```python
from build123d import *
from build123d.topology import SkipClean

# Parameters (mm, degrees)
SKETCH2_W                           = 45
SKETCH2_H                           = 59.874368671
MAIN_EXTRUDE_DEPTH                  = 3
BOWDEN_HOLE_D                       = 4
SKETCH7_R                           = 3.5
SPACER_PILLARS_DEPTH                = 22.1
TOP_THREADS_D                       = 2.5
TOP_THREADS_DEPTH                   = 10
TOP_THREADS_TIP                     = 0.751075774
TOP_THROUGH_HOLE_D                  = 3.2
SKETCH28_R                          = 12.7
SKETCH28_R_2                        = 2
BOSS_EXTRUDE3_DEPTH                 = 2
CHUBE_MOUNTING_D                    = 3.2
CHUBE_MOUNTING_CSINK_D              = 6.72
CHUBE_MOUNTING_CSINK_ANGLE          = 90
BOSS_EXTRUDE4_DEPTH                 = 2
CARRIAGE_HOLES_D                    = 3.2
CARRIAGE_HOLES_DEPTH                = 8
CARRIAGE_HOLES_CSINK_D              = 6.72
CARRIAGE_HOLES_CSINK_ANGLE          = 90
CARRIAGE_HOLES_TIP                  = 0.96137699
BEACON_SLM_SUPPORT_HOLES_AT_2_COUNT = 2
BEACON_SLM_SUPPORT_HOLES_AT_2_PITCH = 24.748737342
BEACON_SLM_SUPPORT_HOLES_AT_3_COUNT = 2
BEACON_SLM_SUPPORT_HOLES_AT_3_PITCH = 24.748737342


with BuildPart() as part:
    # Sketch2 → Main Extrude (new body)
    with BuildSketch(Plane(origin=(0, 0, 0), x_dir=(1, 0, 0), z_dir=(0, 1, 0))):
        with Locations((-6.625631329, 14.062815665)):
            Rectangle(SKETCH2_W, SKETCH2_H)
    extrude(amount=MAIN_EXTRUDE_DEPTH)

    # Bowden Hole (through all)
    with Locations(Plane(origin=(0, 3, 0), x_dir=(1, 0, 0), z_dir=(0, 1, 0))):
        with Locations((0, 0)):
            Hole(BOWDEN_HOLE_D / 2)

    # Sketch7 → Spacer Pillars (add)
    with BuildSketch(Plane(origin=(0, 3, 0), x_dir=(1, 0, 0), z_dir=(0, 1, 0))):
        with Locations(Location((-25.625631329, 40.5, 0), (0, 0, 90))):
            Circle(SKETCH7_R)
        with Locations(Location((12.374368671, 40.5, 0), (0, 0, 90))):
            Circle(SKETCH7_R)
        with Locations(Location((-19.761284896, -2.993325275, 0), (0, 0, 90))):
            Circle(SKETCH7_R)
        with Locations(Location((12.374368671, -12.374368671, 0), (0, 0, 270))):
            Circle(SKETCH7_R)
    extrude(amount=SPACER_PILLARS_DEPTH)

    # Top Threads
    with Locations(Plane(origin=(0, 25.1, 0), x_dir=(1, 0, 0), z_dir=(0, 1, 0))):
        with Locations((12.374368671, 40.5), (-19.761284896, -2.993325275), (-25.625631329, 40.5)):
            Hole(TOP_THREADS_D / 2, depth=TOP_THREADS_DEPTH)
            with Locations((0, 0, -(TOP_THREADS_DEPTH + TOP_THREADS_TIP / 2))):  # 118° drill point
                Cone(0, TOP_THREADS_D / 2, TOP_THREADS_TIP, mode=Mode.SUBTRACT)

    # Top Through Hole (through all)
    with Locations(Plane(origin=(0, 25.1, 0), x_dir=(1, 0, 0), z_dir=(0, 1, 0))):
        with Locations((12.374368671, -12.374368671)):
            Hole(TOP_THROUGH_HOLE_D / 2)

    # Sketch28 → Boss-Extrude3 (add)
    with SkipClean():  # the faces are left unmerged after this step: merging them gives an invalid solid
        with BuildSketch(Plane(origin=(0, 3, 0), x_dir=(1, 0, 0), z_dir=(0, 1, 0))):
            with Locations(Location((0, 0, 0), (0, 0, 90))):
                Circle(SKETCH28_R)
            with Locations(Location((0, 0, 0), (0, 0, 270))):
                Circle(SKETCH28_R_2, mode=Mode.SUBTRACT)
        extrude(amount=BOSS_EXTRUDE3_DEPTH)

    # Chube Mounting (through all)
    with Locations(Plane(origin=(0, 5, 0), x_dir=(1, 0, 0), z_dir=(0, 1, 0))):
        with Locations((-4.5, 7.794228634), (4.5, 7.794228634), (9, 0), (4.5, -7.794228634), (-4.5, -7.794228634), (-9, 0)):
            CounterSinkHole(CHUBE_MOUNTING_D / 2, CHUBE_MOUNTING_CSINK_D / 2, counter_sink_angle=CHUBE_MOUNTING_CSINK_ANGLE)

    # Sketch29 → Boss-Extrude4 (add)
    with SkipClean():  # the faces are left unmerged after this step: merging them gives an invalid solid
        with BuildSketch(Plane(origin=(0, 3, 0), x_dir=(1, 0, 0), z_dir=(0, 1, 0))):
            with BuildLine():
                Line((-17.181637577, 40.5), (-17.181637577, 20.5))
                ThreePointArc((-17.181637577, 20.5), (-16.156511311, 18.025126266), (-13.681637577, 17))
                Line((-13.681637577, 17), (1.318362423, 17))
                ThreePointArc((1.318362423, 17), (3.793236157, 18.025126266), (4.818362423, 20.5))
                Line((4.818362423, 20.5), (4.818362423, 40.5))
                ThreePointArc((4.818362423, 40.5), (3.793236157, 42.974873734), (1.318362423, 44))
                Line((1.318362423, 44), (-13.681637577, 44))
                ThreePointArc((-13.681637577, 44), (-16.156511311, 42.974873734), (-17.181637577, 40.5))
            make_face()
        extrude(amount=BOSS_EXTRUDE4_DEPTH)

    # Carriage Holes
    with Locations(Plane(origin=(0, 5, 0), x_dir=(1, 0, 0), z_dir=(0, 1, 0))):
        with Locations((1.318362423, 40.5), (1.318362423, 20.5), (-13.681637577, 20.5), (-13.681637577, 40.5)):
            CounterSinkHole(CARRIAGE_HOLES_D / 2, CARRIAGE_HOLES_CSINK_D / 2, depth=CARRIAGE_HOLES_DEPTH, counter_sink_angle=CARRIAGE_HOLES_CSINK_ANGLE)
            with Locations((0, 0, -(CARRIAGE_HOLES_DEPTH + CARRIAGE_HOLES_TIP / 2))):  # 118° drill point
                Cone(0, CARRIAGE_HOLES_D / 2, CARRIAGE_HOLES_TIP, mode=Mode.SUBTRACT)

    # Sketch25 → Beacon SLM Support Holes (revolve, cut)
    with SkipClean():  # the faces are left unmerged after this step: merging them gives an invalid solid
        with BuildSketch(Plane(origin=(-12.374368671, 3, -12.374368671), x_dir=(0, 0, 1), z_dir=(1, 0, 0))):
            Polygon((0, 0), (0, 3), (1.6, 3), (1.6, 1.76), (3.36, 0), align=None)
        beacon_slm_support_holes = revolve(axis=Axis((-12.374368671, 9.35, -12.374368671), (0, -1, 0)), mode=Mode.SUBTRACT)

    # Beacon SLM Support Holes at 2: Beacon SLM Support Holes ×2
    with SkipClean():  # the faces are left unmerged after this step: merging them gives an invalid solid
        with Locations(*[(i * BEACON_SLM_SUPPORT_HOLES_AT_2_PITCH, 0, 0) for i in range(1, BEACON_SLM_SUPPORT_HOLES_AT_2_COUNT)]):
            add(beacon_slm_support_holes, mode=Mode.SUBTRACT)

    # Beacon SLM Support Holes at 3: Beacon SLM Support Holes ×2
    with SkipClean():  # the faces are left unmerged after this step: merging them gives an invalid solid
        with Locations(*[(0, 0, i * BEACON_SLM_SUPPORT_HOLES_AT_3_PITCH) for i in range(1, BEACON_SLM_SUPPORT_HOLES_AT_3_COUNT)]):
            add(beacon_slm_support_holes, mode=Mode.SUBTRACT)


solid = part.part
```
Here's how the part is built. I have some questions about the finished solid (model axes, mm). A direction names the side the tool comes from. Give positions to 0.01 mm unless a question says otherwise; leave off trailing zeros. Order: outer loops, then holes, each group sorted by start corner. A loop starts at its lowest first (then second) coordinate and runs counter-clockwise, first axis right, second up. Notation, with made-up numbers: (53, 60) - (80, 60) arc R3 ccw to (80, 65) - close; hole circle Ø4 at (-1.5, 37). An arc over 180 degrees is marked (long way). Answer as a JSON object with one key per item and string values. Group by question number.
Item 1: If we section it at A-A on x = -4.5: Please give me the cut outline in (y, z).
Item 2: For P1, Ø3.5, axis at x = 0, z = 0, coming from the +Y side; P2, Ø5, axis at x = 1.32, z = -20.5, coming from the +Y side; P3, Ø5, axis at x = 1.5, z = -18, coming from the -Y side; P4, Ø1, axis at y = 4.5, z = -26.5, coming from the -X side, each with a flat end and sliding along its axis, tell me the tip position at first contact or that it passes through.
Item 3: Please list where these lines run through material, in increasing order: probe 1 along X at (y, z) = (18.5, -40.5); probe 2 along Z at (x, y) = (-4.5, 0.8); probe 3 along Y at (x, z) = (-21, -38).
Item 4: If we mould it in two halves opening along X, with no side actions, what happens to faces 3 (the cylindrical face through (-16.18, 3.99, -18.05)), 4 (the cylindrical face through (-13.723, 0.629, 13.235)), 5 (the flat face through (15.874, 1, -14)), 6 (the conical face through (12.35, 14.48, -40.72))? For each: pulls with the +X half, pulls with the -X half, needs draft (parallel to the pull), parting line crosses it, or undercut.
Item 5: Which directions (+Z, -Z, +X, -X, +Y, -Y) give clear straight access to the entire face, cutting with the end or side of a thin tool? Please do faces 1 (the cylindrical face through (13.43, 13.9, 15.71)), 2 (the cylindrical face through (-4.29, 1.6, -9.38)).
Item 6: If we section it at B-B on y = 8.5: Please give me the cut outline in (x, z), and give its area (3 significant figures).
Item 7: If we section it at C-C on z = -34: Please give me the cut outline in (x, y), and give its area (3 significant figures).
Result set:
{
 "1": {"outline": "(0, -44) - (5, -44) - (5, -17) - (3, -17) - (3, -11.88) - (5, -11.88) - (5, -11.15) - (3.24, -9.39) - (0, -9.39) - close; (0, -6.19) - (3.24, -6.19) - (5, -4.43) - (5, 4.43) - (3.24, 6.19) - (0, 6.19) - close; (0, 9.39) - (3.24, 9.39) - (5, 11.15) - (5, 11.88) - (3, 11.88) - (3, 15.87) - (0, 15.87) - close"},
 "2": {"P1": "through", "P2": "y = 4.14", "P3": "y = 0", "P4": "x = -17.18"},
 "3": {"probe 1": "-29.13 to -26.88, -24.38 to -22.13, 8.87 to 11.12, 13.62 to 15.87", "probe 2": "-44 to -9.39, -6.19 to 6.19, 9.39 to 15.87", "probe 3": "0 to 3"},
 "4": {"face 3": "pulls with the -X half", "face 4": "undercut", "face 5": "pulls with the +X half", "face 6": "undercut"},
 "5": {"face 1": "+Y", "face 2": "+Y, -Y"},
 "6": {"outline": "circle Ø7 at (-25.63, -40.5); circle Ø7 at (-19.76, 2.99); circle Ø7 at (12.37, -40.5); circle Ø7 at (12.37, 12.37); hole circle Ø3.2 at (12.37, 12.37)", "area": "146 mm²"},
 "7": {"outline": "(-29.13, 0) - (15.87, 0) - (15.87, 3) - (4.82, 3) - (4.82, 5) - (-17.18, 5) - (-17.18, 3) - (-29.13, 3) - close", "area": "179 mm²"}
}
